For this review, take the finished solid that the model builds, in its own axes (mm). Face numbers are marked on the shaded views. A direction names the side the tool comes from. Coordinates: 2 decimals unless noted, no trailing zeros. Write each loop counter-clockwise with the first axis right and the second up, starting at its lowest first coordinate (ties: lowest second). Pieces come first, ordered by that corner, then holes.
1) To check wall thickness, follow line 1 along X through (y, z) = (0.45, 0); line 2 along X through (y, z) = (1.35, 1.25); line 3 along Z through (x, y) = (-0.75, 1.5). State the ranges of each line that lie inside material, in increasing order.
2) For the marked faces 4, 5 and 6, list the 3-axis set-ups (+Z, -Z, +X, -X, +Y, -Y) from which the entire face can be reached by the end or side of a thin tool; tool diameter is ignored.
3) We need section C-C on x = 0. Write out the cut boundary in (y, z), then the cut area to 3 significant figures.
4) Insertion check: P1, Ø1, axis at y = 1, z = 3.5, coming from the -X side; P2, Ø0.5, axis at y = 0.5, z = 0.5, coming from the +X side. Each pin has a flat end and moves straight along its axis. Give the tip position at first contact, or say it passes through.
5) We need section B-B on y = 0.6. Write out the cut boundary in (x, z).
6) Mouldability with a two-part tool opening along Z and no side actions: class the marked faces 1, 2 and 3 as pulls with the +Z half, pulls with the -Z half, needs draft (parallel to the pull), parting line crosses it, or undercut.
7) We need section D-D on z = 1.75. Write out the cut boundary in (x, y), then the cut area to 3 significant figures.
8) We need section A-A on z = 0. Write out the cut boundary in (x, y), then the cut area to 3 significant figures.
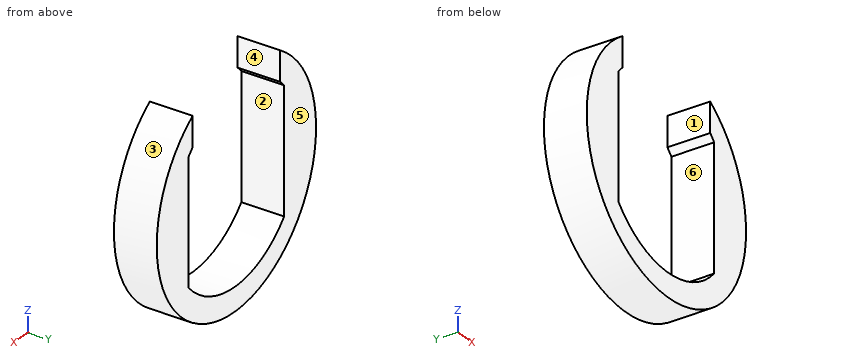
from build123d import *

# Parameters (mm, degrees)
SKETCH1_R           = 5
BOSS_EXTRUDE1_DEPTH = 1.8
CUT_EXTRUDE1_DEPTH  = 2.8


with BuildPart() as part:
    # Sketch1 → Boss-Extrude1 (new body)
    with BuildSketch(Plane(origin=(0, 0, 0), x_dir=(1, 0, 0), z_dir=(0, 1, 0))):
        Circle(SKETCH1_R)
    extrude(amount=BOSS_EXTRUDE1_DEPTH)

    # Sketch2 → Cut-Extrude1 (cut, through all)
    with BuildSketch(Plane(origin=(0, 1.8, 0), x_dir=(1, 0, 0), z_dir=(0, 1, 0))):
        with BuildLine():
            Line((-3, 2.645751311), (-3, -2.645751311))
            ThreePointArc((-3, -2.645751311), (-2.877914777, -2.778058051), (-2.75, -2.90473751))
            Line((-2.75, -2.90473751), (-2.75, -4.175823272))
            ThreePointArc((-2.75, -4.175823272), (0, -5), (2.75, -4.175823272))
            Line((2.75, -4.175823272), (2.75, -2.90473751))
            ThreePointArc((2.75, -2.90473751), (2.877914777, -2.778058051), (3, -2.645751311))
            Line((3, -2.645751311), (3, 2.645751311))
            ThreePointArc((3, 2.645751311), (0, 4), (-3, 2.645751311))
        make_face()
    extrude(amount=-CUT_EXTRUDE1_DEPTH, mode=Mode.SUBTRACT)


solid = part.part
Result:
1. line 1: x = -5 to -3, 3 to 5
1. line 2: x = -4.84 to -3, 3 to 4.84
1. line 3: z = -4.94 to -3.93
2. face 4: +Z, +Y, -Y
2. face 5: +Z, -Z, +X, -X, +Y
2. face 6: +Y, -Y
3. outline: (0, -5) - (1.8, -5) - (1.8, -4) - (0, -4) - close
3. area: 1.80 mm2
4. P1: stops at x = -4
4. P2: stops at x = 4.99
5. outline: (-3, -2.65) - (-3, 2.65) arc R4 cw to (-2.75, 2.9) - (-2.75, 4.18) arc R5 ccw (long way) to (2.75, 4.18) - (2.75, 2.9) arc R4 cw to (3, 2.65) - (3, -2.65) arc R4 cw to start
6. face 1: needs draft
6. face 2: undercut
6. face 3: parting line crosses it
7. outline: (-4.68, 0) - (-3, 0) - (-3, 1.8) - (-4.68, 1.8) - close; (3, 0) - (4.68, 0) - (4.68, 1.8) - (3, 1.8) - close
7. area: 6.06 mm2
8. outline: (-5, 0) - (-3, 0) - (-3, 1.8) - (-5, 1.8) - close; (3, 0) - (5, 0) - (5, 1.8) - (3, 1.8) - close
8. area: 7.20 mm2
